For this review, use the dimensioned drawing (mm, ordinates from the lowest corner) and the shaded views. A direction names the side the tool comes from. Round coordinates to 2 decimals unless told otherwise and drop trailing zeros. Write each loop counter-clockwise with the first axis right and the second up, starting at its lowest first coordinate (ties: lowest second). Pieces come first, ordered by that corner, then holes. Notation, with made-up numbers: (-19, -9.75) -> (-11, -9.75) arc R28 ccw to (-11, 25.25) -> close; hole circle Ø8 at (28, -1). An arc over 180 degrees is marked (long way). Write each question's results on one line, items separated by ' | '. Start each with the question number.
Item 1: The part is to be moulded in two halves that separate along X. For the marked faces 1, 2 and 3, say which applies: +X half, -X half, draft (parallel to the pull), parting line (faces both ways), or undercut.
Item 2: To check wall thickness, follow line 1 along X through (y, z) = (10.5, 2.5); line 2 along Y through (x, z) = (48.95, 20); line 3 along Y through (x, z) = (46, 19.5). State the ranges of each line that lie inside material, in increasing order.
Item 3: Tool access review of the marked faces 4 and 5: name each direction out of +Z, -Z, +X, -X, +Y, -Y from which nothing blocks a thin tool from reaching the whole face with its end or side.
Item 4: Clearance check with a flat-ended pin moving along its axis: pin 1 (12 mm diameter, centred on x = 27, z = 11.5, fed in from +Y). State where the tip first meets the part, or that it passes through.
Item 5: Add section A-A (y = 6). State the section outline as (x, z) points.
Item 6: Add section C-C (y = 32.5). State the section outline as (x, z) points.
Item 7: Add section D-D (z = 5). State the section outline as (x, y) points, plus the area to 3 significant figures.
Item 8: Add section B-B (z = 20). State the section outline as (x, y) points.
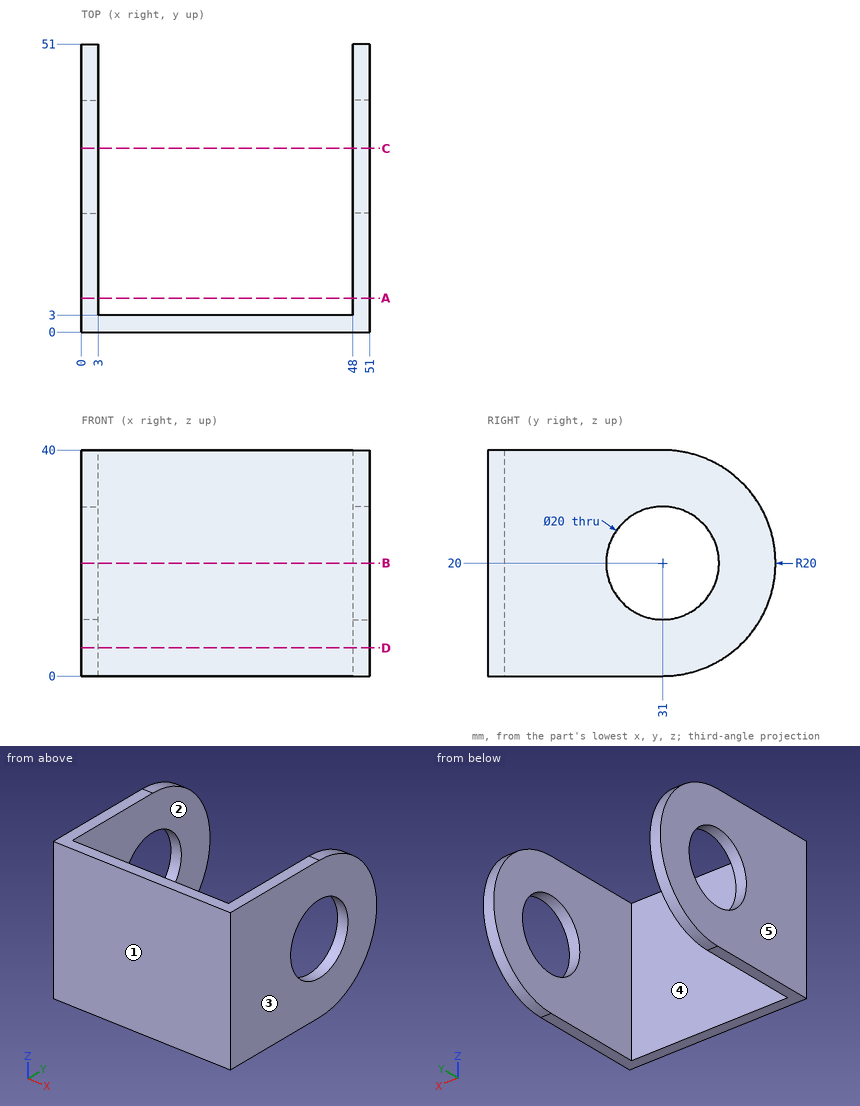
Responses:
1) face 1: draft | face 2: undercut | face 3: +X half
2) line 1: x = 0 to 3, 48 to 51 | line 2: y = 0 to 21, 41 to 51 | line 3: y = 0 to 3
3) face 4: +Z, -Z, +Y | face 5: +Z, -Z, -X, +Y, -Y
4) pin 1: stops at y = 3
5) outline: (0, 0) -> (3, 0) -> (3, 40) -> (0, 40) -> close; (48, 0) -> (51, 0) -> (51, 40) -> (48, 40) -> close
6) outline: (0, 0.06) -> (3, 0.06) -> (3, 10.11) -> (0, 10.11) -> close; (0, 29.89) -> (3, 29.89) -> (3, 39.94) -> (0, 39.94) -> close; (48, 0.06) -> (51, 0.06) -> (51, 10.11) -> (48, 10.11) -> close; (48, 29.89) -> (51, 29.89) -> (51, 39.94) -> (48, 39.94) -> close
7) outline: (0, 0) -> (51, 0) -> (51, 44.23) -> (48, 44.23) -> (48, 3) -> (3, 3) -> (3, 44.23) -> (0, 44.23) -> close | area: 400 mm^2
8) outline: (0, 0) -> (51, 0) -> (51, 21) -> (48, 21) -> (48, 3) -> (3, 3) -> (3, 21) -> (0, 21) -> close; (0, 41) -> (3, 41) -> (3, 51) -> (0, 51) -> close; (48, 41) -> (51, 41) -> (51, 51) -> (48, 51) -> close
